Read the model definition and answer for the solid it produces. Units are mm, in the model's axes. A direction names the side the tool comes from. Coordinates: 2 decimals unless noted, no trailing zeros. Order: outer loops, then holes, each group sorted by start corner. A loop starts at its lowest first (then second) coordinate and runs counter-clockwise, first axis right, second up. Notation, with made-up numbers: M 24,79 L 40,79 A8 ccw 40,94 Z; hole C -1,29 d11. An arc over 180 degrees is marked long. Put each result on its own line as item: value.
from build123d import *

# Parameters (mm, degrees)
F1_DEPTH = 25.4
F2_W     = 25.4
F2_H     = 12.7
F3_DEPTH = 3.175
F4_DEPTH = 76.2
F5_START = 76.2
F5_DEPTH = 3.175
F6_DEPTH = 3.175
F8_DEPTH = 25.4


# Not quite as in the source:
# - a feature names something its author has since deleted; it is built from what else it names


with BuildPart() as f1:
    # F0 (on Front) → F1 (new body)
    with BuildSketch(Plane.XZ):
        with BuildLine():
            Line((5.55625, 0), (0, 0))
            Line((0, 0), (0, -31.75))
            Line((0, -31.75), (9.525, -31.75))
            Line((9.525, -31.75), (9.525, -10.5061289571))
            ThreePointArc((9.525, -10.5061289571), (8.73125, -8.73125), (9.525, -6.9563710429))
            Line((9.525, -6.9563710429), (9.525, -3.175))
            Line((9.525, -3.175), (11.1125, -3.175))
            Line((11.1125, -3.175), (12.7, -3.175))
            Line((12.7, -3.175), (12.7, -6.35))
            Line((12.7, -6.35), (12.7, -6.9563710429))
            ThreePointArc((12.7, -6.9563710429), (13.49375, -8.73125), (12.7, -10.5061289571))
            Line((12.7, -10.5061289571), (12.7, -28.575))
            Line((12.7, -28.575), (12.7, -31.75))
            Line((12.7, -31.75), (19.05, -31.75))
            Line((19.05, -31.75), (19.05, 0))
            Line((19.05, 0), (16.66875, 0))
            Line((16.66875, 0), (14.2875, 2.6339585893))
            ThreePointArc((14.2875, 2.6339585893), (11.1125, 5.8089585893), (7.9375, 2.6339585893))
            Line((7.9375, 2.6339585893), (5.55625, 0))
        make_face()
        with BuildLine():
            Line((12.7, 0), (11.1125, 0))
            Line((11.1125, 0), (9.525, 0))
            Line((9.525, 0), (9.525, 2.6339585893))
            ThreePointArc((9.525, 2.6339585893), (11.1125, 4.2214585893), (12.7, 2.6339585893))
            Line((12.7, 2.6339585893), (12.7, 0))
        make_face(mode=Mode.SUBTRACT)
    extrude(amount=F1_DEPTH)

    # F2 (on face) → F3 (join)
    with BuildSketch(Plane(origin=(0, 0, 0), x_dir=(0, -1, 0), z_dir=(-1, 0, 0))):
        with BuildLine():
            ThreePointArc((0, 15.186421298), (12.7, 17.6824416941), (25.4, 15.186421298))
            Line((25.4, 15.186421298), (25.4, 20.0460244843))
            ThreePointArc((25.4, 20.0460244843), (12.7, 22.225), (0, 20.0460244843))
            Line((0, 20.0460244843), (0, 15.186421298))
        make_face()
        with BuildLine():
            Line((0, 0), (25.4, 0))
            Line((25.4, 0), (25.4, 15.186421298))
            ThreePointArc((25.4, 15.186421298), (12.7, 17.6824416941), (0, 15.186421298))
            Line((0, 15.186421298), (0, 0))
        make_face()
        with BuildLine():
            Line((0, -31.75), (0, -46.936421298))
            ThreePointArc((0, -46.936421298), (12.7, -49.4324416941), (25.4, -46.936421298))
            Line((25.4, -46.936421298), (25.4, -31.75))
            Line((25.4, -31.75), (0, -31.75))
        make_face()
        with BuildLine():
            Line((0, -46.936421298), (0, -51.7960244843))
            ThreePointArc((0, -51.7960244843), (12.7, -53.975), (25.4, -51.7960244843))
            Line((25.4, -51.7960244843), (25.4, -46.936421298))
            ThreePointArc((25.4, -46.936421298), (12.7, -49.4324416941), (0, -46.936421298))
        make_face()
        with Locations((12.7, -25.4)):
            Rectangle(F2_W, F2_H)
        with Locations((12.7, -6.35)):
            Rectangle(F2_W, F2_H)
        Polygon((0, -15.875), (0, -19.05), (25.4, -19.05), (25.4, -12.7), (0, -12.7), align=None)
    extrude(amount=F3_DEPTH)

    # F2 (on face) → F4 (join)
    with BuildSketch(Plane(origin=(0, 0, 0), x_dir=(0, -1, 0), z_dir=(-1, 0, 0))):
        with BuildLine():
            ThreePointArc((0, 15.186421298), (12.7, 17.6824416941), (25.4, 15.186421298))
            Line((25.4, 15.186421298), (25.4, 20.0460244843))
            ThreePointArc((25.4, 20.0460244843), (12.7, 22.225), (0, 20.0460244843))
            Line((0, 20.0460244843), (0, 15.186421298))
        make_face()
        with BuildLine():
            Line((0, -46.936421298), (0, -51.7960244843))
            ThreePointArc((0, -51.7960244843), (12.7, -53.975), (25.4, -51.7960244843))
            Line((25.4, -51.7960244843), (25.4, -46.936421298))
            ThreePointArc((25.4, -46.936421298), (12.7, -49.4324416941), (0, -46.936421298))
        make_face()
    extrude(amount=F4_DEPTH)

    # F2 (on face) → F5 (join)
    with BuildSketch(Plane(origin=(0, 0, 0), x_dir=(0, -1, 0), z_dir=(-1, 0, 0)).offset(F5_START)):
        with BuildLine():
            ThreePointArc((25.4, -51.7960244843), (12.7, -53.975), (0, -51.7960244843))
            Line((0, -51.7960244843), (0, -54.4783297054))
            ThreePointArc((0, -54.4783297054), (12.7, -56.5137384689), (25.4, -54.4783297054))
            Line((25.4, -54.4783297054), (25.4, -51.7960244843))
        make_face()
        with BuildLine():
            Line((0, -46.936421298), (0, -51.7960244843))
            ThreePointArc((0, -51.7960244843), (12.7, -53.975), (25.4, -51.7960244843))
            Line((25.4, -51.7960244843), (25.4, -46.936421298))
            ThreePointArc((25.4, -46.936421298), (12.7, -49.4324416941), (0, -46.936421298))
        make_face()
        with BuildLine():
            Line((0, -31.75), (0, -46.936421298))
            ThreePointArc((0, -46.936421298), (12.7, -49.4324416941), (25.4, -46.936421298))
            Line((25.4, -46.936421298), (25.4, -31.75))
            Line((25.4, -31.75), (0, -31.75))
        make_face()
        with Locations((12.7, -25.4)):
            Rectangle(F2_W, F2_H)
        with Locations((12.7, -6.35)):
            Rectangle(F2_W, F2_H)
        with BuildLine():
            Line((0, 0), (25.4, 0))
            Line((25.4, 0), (25.4, 15.186421298))
            ThreePointArc((25.4, 15.186421298), (12.7, 17.6824416941), (0, 15.186421298))
            Line((0, 15.186421298), (0, 0))
        make_face()
        with BuildLine():
            ThreePointArc((0, 15.186421298), (12.7, 17.6824416941), (25.4, 15.186421298))
            Line((25.4, 15.186421298), (25.4, 20.0460244843))
            ThreePointArc((25.4, 20.0460244843), (12.7, 22.225), (0, 20.0460244843))
            Line((0, 20.0460244843), (0, 15.186421298))
        make_face()
        with BuildLine():
            ThreePointArc((0, 20.0460244843), (12.7, 22.225), (25.4, 20.0460244843))
            Line((25.4, 20.0460244843), (25.4, 22.7283297054))
            ThreePointArc((25.4, 22.7283297054), (12.7, 24.7637384689), (0, 22.7283297054))
            Line((0, 22.7283297054), (0, 20.0460244843))
        make_face()
    extrude(amount=F5_DEPTH)

    # F2 (on face) → F6 (join)
    with BuildSketch(Plane(origin=(0, 0, 0), x_dir=(0, -1, 0), z_dir=(-1, 0, 0))):
        with BuildLine():
            ThreePointArc((0, 20.0460244843), (12.7, 22.225), (25.4, 20.0460244843))
            Line((25.4, 20.0460244843), (25.4, 22.7283297054))
            ThreePointArc((25.4, 22.7283297054), (12.7, 24.7637384689), (0, 22.7283297054))
            Line((0, 22.7283297054), (0, 20.0460244843))
        make_face()
        with BuildLine():
            ThreePointArc((0, 15.186421298), (12.7, 17.6824416941), (25.4, 15.186421298))
            Line((25.4, 15.186421298), (25.4, 20.0460244843))
            ThreePointArc((25.4, 20.0460244843), (12.7, 22.225), (0, 20.0460244843))
            Line((0, 20.0460244843), (0, 15.186421298))
        make_face()
        with BuildLine():
            Line((0, -46.936421298), (0, -51.7960244843))
            ThreePointArc((0, -51.7960244843), (12.7, -53.975), (25.4, -51.7960244843))
            Line((25.4, -51.7960244843), (25.4, -46.936421298))
            ThreePointArc((25.4, -46.936421298), (12.7, -49.4324416941), (0, -46.936421298))
        make_face()
        with BuildLine():
            ThreePointArc((25.4, -51.7960244843), (12.7, -53.975), (0, -51.7960244843))
            Line((0, -51.7960244843), (0, -54.4783297054))
            ThreePointArc((0, -54.4783297054), (12.7, -56.5137384689), (25.4, -54.4783297054))
            Line((25.4, -54.4783297054), (25.4, -51.7960244843))
        make_face()
    extrude(amount=-F6_DEPTH)

    # F7 (on face) → F8 (join)
    with BuildSketch(Plane(origin=(0, 0, 0), x_dir=(-1, 0, 0), z_dir=(0, 1, 0))):
        with BuildLine():
            ThreePointArc((72.300083342, -12.7020545776), (72.4126137623, -12.7000004406), (72.5251462844, -12.7019360086))
            Line((72.5251462844, -12.7019360086), (76.2, -12.7))
            Line((76.2, -12.7), (76.2, -9.5260270395))
            Line((76.2, -9.5260270395), (72.5284895273, -9.5260270395))
            Line((72.5284895273, -9.5260270395), (72.300083342, -9.5260270395))
            ThreePointArc((72.300083342, -9.5260270395), (66.0645431997, -15.9321038554), (72.4142864347, -22.225))
            Line((72.4142864347, -22.225), (76.2, -22.225))
            Line((76.2, -22.225), (76.2, -19.05))
            Line((76.2, -19.05), (72.4142864347, -19.05))
            ThreePointArc((72.4142864347, -19.05), (69.2398001206, -15.9321107863), (72.300083342, -12.7020545776))
        make_face()
    extrude(amount=-F8_DEPTH)

    # F9: sweep along a path in F9_path
    with BuildLine(Plane(origin=(-79.375, 0, 22.7283297054), x_dir=(0, 0, -1), z_dir=(-1, 0, 0))) as f9_path:
        ThreePointArc((0, 0), (-2.0354087635, 12.7), (0, 25.4))
    # F7 (on face) → F9 (sweep, cut)
    with BuildSketch(Plane(origin=(0, 0, 0), x_dir=(-1, 0, 0), z_dir=(0, 1, 0))):
        with BuildLine():
            ThreePointArc((76.2, 21.3871770949), (77.7875, 22.7182272858), (79.375, 21.3871770949))
            Line((79.375, 21.3871770949), (79.375, 22.7283297054))
            Line((79.375, 22.7283297054), (77.7875, 22.7283297054))
            Line((77.7875, 22.7283297054), (76.2, 22.7283297054))
            Line((76.2, 22.7283297054), (76.2, 21.3871770949))
        make_face()
    sweep(path=f9_path.line, mode=Mode.SUBTRACT)


solid = f1.part
Q1. Find section C-C on z = -21. Write down the section's boundary in (x, y) (3 decimals), plus the area to 3 significant figures.
Answers below:
outline: M -79.375,-25.4 L -68.665,-25.4 L -68.665,0 L -79.375,0 Z; M -3.175,-25.4 L 9.525,-25.4 L 9.525,0 L -3.175,0 Z; M 12.7,-25.4 L 19.05,-25.4 L 19.05,0 L 12.7,0 Z
area: 756 mm^2
Q2. A tool of negligible diameter and unlimited length cuts with its end or side. For faces 4 (the face through (1.57, -12.52, 17.68)), 5 (the face through (5, -13, -31.75)), 6 (the face through (-74, -13, -9.526)), 7 (the face through (0, -13, 23)), from which of +Z, -Z, +X, -X, +Y, -Y can it reach the whole face along a straight path? Write none if from no direction.
Answers below:
face 4: +X
face 5: +X, +Y, -Y
face 6: +Y, -Y
face 7: +Z
Q3. Find section B-B on x = -51.5. Write down the section's boundary in (y, z) (3 decimals), plus the area to 3 significant figures.
Answers below:
outline: M -25.4,-51.796 A38.1 ccw 0,-51.796 L 0,-46.936 A33.557 cw -25.4,-46.936 Z; M -25.4,15.186 A33.557 cw 0,15.186 L 0,20.046 A38.1 ccw -25.4,20.046 Z
area: 236 mm^2
Q4. Consider line 1 along X through (y, z) = (-16.5, -22.5) (3 decimals); line 2 along X through (y, z) = (-12.5, 14.5) (3 decimals); line 3 along X through (y, z) = (-2, -10) (3 decimals). Determine where each line is inside the solid, lowest interval first.
Answers below:
line 1: x = -79.375 to -76.2, -3.175 to 9.525, 12.7 to 19.05
line 2: x = -79.375 to -76.2, -3.175 to 0
line 3: x = -79.375 to -70.005, -3.175 to 9.097, 13.128 to 19.05
Q5. For a pull along Z with two mould halves and no side action, classify faces 1 (the face through (1.565, -12.519, -56.513)), 2 (the face through (9.525, -13, -5)), 3 (the face through (12.7, -13, 1)) as +Z half, -Z half, draft (parallel to the pull), parting line (faces both ways), or undercut.
Answers below:
face 1: -Z half
face 2: draft
face 3: undercut
Q6. Find section D-D on y = -6. Give the number of separate pieces and of enclosed holes in the cut face, plus the area to 3 significant figures.
Answers below:
separate pieces: 1
enclosed holes: 2
area: 1,800 mm^2
Q7. Given pin 1 (4.5 mm diameter, centred on x = -73.5, y = -15, fed in from +Z); pin 2 (1.9 mm diameter, centred on x = 17.5, y = -12.5, fed in from +Z); pin 3 (1.7 mm diameter, centred on y = -17.5, z = 22, fed in from +X) (3 decimals), each flat-ended and moving along its own axis, determine where each tip first touches the part or whether it passes through.
Answers below:
pin 1: stops at z = 22.22
pin 2: stops at z = 0.13
pin 3: stops at x = 3.175
Q8. Find section A-A on z = -1.5. Write down the section's boundary in (x, y) (3 decimals), plus the area to 3 significant figures.
Answers below:
outline: M -79.375,-25.4 L -76.2,-25.4 L -76.2,0 L -79.375,0 Z; M -3.175,-25.4 L 19.05,-25.4 L 19.05,0 L -3.175,0 Z
area: 645 mm^2
